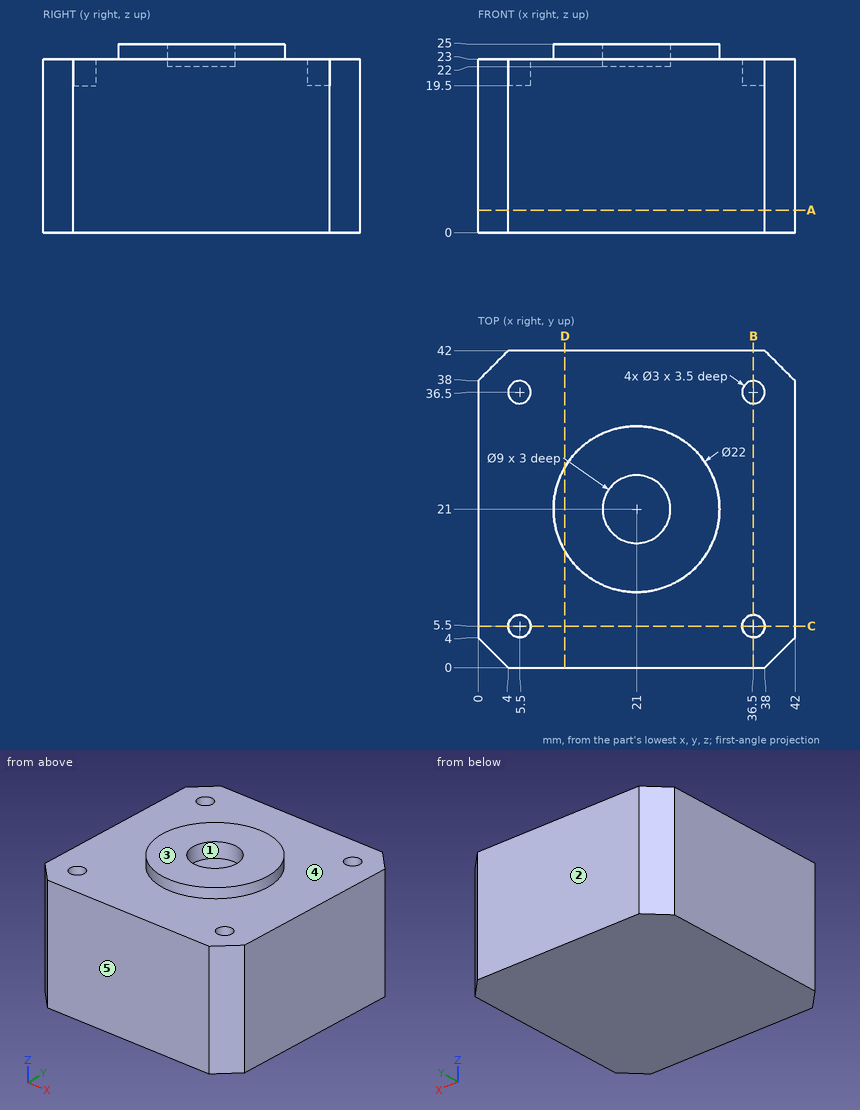
Answer from the drawing. Dimensions are ordinates in mm from the lowest x, y and z of the part. A direction names the side the tool comes from. Coordinates: 2 decimals unless noted, no trailing zeros. Write each loop counter-clockwise with the first axis right and the second up, starting at its lowest first coordinate (ties: lowest second). Pieces come first, ordered by that corner, then holes. Notation, with made-up numbers: (27.5, 24) - (67.5, 24) arc R30 cw to (67.5, 59) - close; hole circle Ø3 at (-0.5, 1.5). An arc over 180 degrees is marked (long way). Answer as CSV lines item,"result".
1. Given P1, Ø1.5, axis at x = 37, y = 5, coming from the +Z side; P2, Ø5, axis at x = 5.5, y = 36.5, coming from the +Z side; P3, Ø2.5, axis at x = 19.5, y = 19.5, coming from the +Z side, each flat-ended and moving along its own axis, determine where each tip first touches the part or whether it passes through.
Computed values:
P1,"stops at z = 19.5"
P2,"stops at z = 23"
P3,"stops at z = 22"
2. A tool of negligible diameter and unlimited length cuts with its end or side. For the marked faces 4 and 5, from which of +Z, -Z, +X, -X, +Y, -Y can it reach the whole face along a straight path? Write none if from no direction.
Computed values:
face 4,"+Z"
face 5,"+Z, -Z, +X, -X, -Y"
3. Find section B-B (x = 36.5). Give the vertices of the cut face in (y, z).
Computed values:
outline,"(0, 0) - (42, 0) - (42, 23) - (38, 23) - (38, 19.5) - (35, 19.5) - (35, 23) - (7, 23) - (7, 19.5) - (4, 19.5) - (4, 23) - (0, 23) - close"
4. Find section A-A (z = 3). Give the vertices of the cut face in (x, y).
Computed values:
outline,"(0, 4) - (4, 0) - (38, 0) - (42, 4) - (42, 38) - (38, 42) - (4, 42) - (0, 38) - close"
5. Find section D-D (x = 11.5). Give the vertices of the cut face in (y, z), plus the area to 3 significant figures.
Computed values:
outline,"(0, 0) - (42, 0) - (42, 23) - (26.55, 23) - (26.55, 25) - (15.45, 25) - (15.45, 23) - (0, 23) - close"
area,"988 mm²"
6. Straight lines are drawn through the part: line 1 (Y direction, x = 5.5, z = 22.1); line 2 (Y direction, x = 21, z = 23.05). For each, find the intervals that lie inside material, in ascending order. Write a range as [from, to].
Computed values:
line 1,"y = [0, 4], [7, 35], [38, 42]"
line 2,"y = [10, 16.5], [25.5, 32]"
7. Determine the mould class of the marked faces 1, 2 and 3 for opening direction Y: +Y half, -Y half, draft (parallel to the pull), parting line (faces both ways), or undercut.
Computed values:
face 1,"undercut"
face 2,"+Y half"
face 3,"draft"
